Geometry: final body of the model. Coordinates: model frame, mm. A direction names the side the tool comes from. Round coordinates to 2 decimals unless told otherwise and drop trailing zeros. Loops run counter-clockwise (first coordinate to the right, second up) from the corner with the lowest first, then second, coordinate; pieces in that order, holes last. Notation, with made-up numbers: (-14, 16.5) - (19, 16.5) arc R25 cw to (19, 51.5) - close; hole circle Ø7 at (-9, 74.5). An arc over 180 degrees is marked (long way). Write item = value, one per line. Start each with the question number.
Item 1: Section D-D (x = -10). Return loops of the section in (y, z) (3 decimals).
Item 2: Section B-B (z = 15.5). Return loops of the section in (x, y) (3 decimals), plus the area to 4 significant figures.
Item 3: Line query: line 1 (Z direction, x = 7, y = 31.2) (3 decimals); line 2 (Z direction, x = 0.7, y = -15.5) (3 decimals); line 3 (Y direction, x = -16.5, z = -9). Output: solid intervals per line, ascending. Write a range as from..to.
Item 4: Draft query along X for faces 4 (the flat face through (25, 30, 0)), 5 (the flat face through (-4, 21, -25)), 6 (the cylindrical face through (-9.648, 30.479, 17.414)). Return one class per face: pulls with the +X half, pulls with the -X half, needs draft (parallel to the pull), parting line crosses it, or undercut.
Item 5: First-contact query: pin 1 (2.5 mm diameter, centred on x = -10, z = 0, fed in from +Y); pin 2 (2 mm diameter, centred on x = 9, z = -0.5, fed in from -Y); pin 3 (3.5 mm diameter, centred on y = -15.5, z = -15.5, fed in from +X); pin 4 (15 mm diameter, centred on y = -7.5, z = 3, fed in from -X). Flat tips, straight axial feed; report the tip coordinate or a pass-through.
Item 6: Access query for faces 1 (the flat face through (-1.5, 14, 0)), 2 (the flat face through (1.5, 3.1, 11.5)), 3 (the cylindrical face through (-0.02, 16.25, -16.94)). Directions: +Z, -Z, +X, -X, +Y, -Y. A direction counts if a zero-diameter tool reaches every point of the face in a straight line with its end or side. Return the directions, or none.
Item 7: Section A-A (y = -15.5). Return loops of the section in (x, z) (3 decimals).
Item 8: Section C-C (y = -2). Return loops of the section in (x, z), plus the area to 3 significant figures.
from build123d import *

# Parameters (mm, degrees)
F0_W     = 51
F0_H     = 50
F0_R     = 1.625
F0_R_2   = 11.5
F1_DEPTH = 1.5
F2_W     = 50
F2_H     = 50
F2_R     = 1.625
F3_DEPTH = 3
F6_DEPTH = 3
F7_DEPTH = 3


with BuildPart() as f1:
    # F0 (on Right) → F1 (new body, symmetric)
    with BuildSketch(Plane.YZ):
        with Locations((3.5, 0)):
            Rectangle(F0_W, F0_H)
        with Locations((-15.5, -15.5)):
            Circle(F0_R, mode=Mode.SUBTRACT)
        with Locations((15.5, -15.5)):
            Circle(F0_R, mode=Mode.SUBTRACT)
        Circle(F0_R_2, mode=Mode.SUBTRACT)
        with Locations((-15.5, 15.5)):
            Circle(F0_R, mode=Mode.SUBTRACT)
        with Locations((15.5, 15.5)):
            Circle(F0_R, mode=Mode.SUBTRACT)
    extrude(amount=F1_DEPTH, both=True)

    # F2 (on face) → F3 (join)
    with BuildSketch(Plane(origin=(0, 29, 0), x_dir=(-1, 0, 0), z_dir=(0, 1, 0))):
        Rectangle(F2_W, F2_H)
        with Locations((-7, 0)):
            Circle(F2_R, mode=Mode.SUBTRACT)
        with Locations((-7, 19)):
            Circle(F2_R, mode=Mode.SUBTRACT)
        with Locations((10, 0)):
            Circle(F2_R, mode=Mode.SUBTRACT)
        with Locations((10, 19)):
            Circle(F2_R, mode=Mode.SUBTRACT)
    extrude(amount=F3_DEPTH)

    # F5 (on face) → F6 (join)
    with BuildSketch(Plane.XY.offset(25)):
        with BuildLine():
            ThreePointArc((-25, 29), (-8.382991, 22.117009), (-1.5, 5.5))
            Line((-1.5, 5.5), (-1.5, 29))
            Line((-1.5, 29), (-25, 29))
        make_face()
    extrude(amount=-F6_DEPTH)

    # F4 (on face) → F7 (join)
    with BuildSketch(Plane(origin=(0, 0, -25), x_dir=(1, 0, 0), z_dir=(0, 0, -1))):
        with BuildLine():
            ThreePointArc((-1.5, -5.5), (-8.382991, -22.117009), (-25, -29))
            Line((-25, -29), (-1.5, -29))
            Line((-1.5, -29), (-1.5, -5.5))
        make_face()
    extrude(amount=-F7_DEPTH)


solid = f1.part
Taken from the geometry:
q1.outline = (23.59, -25) - (32, -25) - (32, -1.625) - (29, -1.625) - (29, -22) - (23.59, -22) - close; (23.59, 22) - (29, 22) - (29, 20.625) - (32, 20.625) - (32, 25) - (23.59, 25) - close; (29, 1.625) - (32, 1.625) - (32, 17.375) - (29, 17.375) - close
q2.outline = (-25, 29) - (-1.5, 29) - (-1.5, 17.125) - (1.5, 17.125) - (1.5, 29) - (25, 29) - (25, 32) - (-25, 32) - close; (-1.5, -22) - (1.5, -22) - (1.5, -17.125) - (-1.5, -17.125) - close; (-1.5, -13.875) - (1.5, -13.875) - (1.5, 13.875) - (-1.5, 13.875) - close
q2.area = 283.5 mm^2
q3.line_1 = -25..-1.625, 1.625..17.375, 20.625..25
q3.line_2 = -25..-17.125, -13.875..13.875, 17.125..25
q3.line_3 = 29..32
q4.face_4 = pulls with the +X half
q4.face_5 = needs draft
q4.face_6 = undercut
q5.pin_1 = through
q5.pin_2 = 29
q5.pin_3 = 1.5
q5.pin_4 = -1.5
q6.face_1 = -X, -Y
q6.face_2 = +Z, -Z, +X, -Y
q6.face_3 = +X, -X
q7.outline = (-1.5, -25) - (1.5, -25) - (1.5, -17.125) - (-1.5, -17.125) - close; (-1.5, -13.875) - (1.5, -13.875) - (1.5, 13.875) - (-1.5, 13.875) - close; (-1.5, 17.125) - (1.5, 17.125) - (1.5, 25) - (-1.5, 25) - close
q8.outline = (-1.5, -25) - (1.5, -25) - (1.5, -11.32) - (-1.5, -11.32) - close; (-1.5, 11.32) - (1.5, 11.32) - (1.5, 25) - (-1.5, 25) - close
q8.area = 82.1 mm^2
